from build123d import *

# Parameters (mm, degrees)
BOSS_EXTRUDE2_DEPTH = 150
SKETCH4_W           = 110
SKETCH4_H           = 150
CUT_EXTRUDE1_DEPTH  = 150
FILLET1_R           = 5
SKETCH5_R           = 17.5
CUT_EXTRUDE2_DEPTH  = 378


with BuildPart() as part:
    # Sketch3 → Boss-Extrude2 (new, symmetric)
    with BuildSketch(Plane.XY):
        with BuildLine():
            Line((0, 0), (150, 0))
            ThreePointArc((150, 0), (188.540496218, 7.5), (150, 15))
            Line((150, 15), (0, 15))
            Line((0, 15), (0, 0))
        make_face()
    extrude(amount=BOSS_EXTRUDE2_DEPTH, both=True)

    # Sketch4 → Cut-Extrude1 (cut, symmetric)
    with BuildSketch(Plane(origin=(0, 0, 0), x_dir=(1, 0, 0), z_dir=(0, 1, 0))):
        with Locations((140, 0)):
            Rectangle(SKETCH4_W, SKETCH4_H)
    extrude(amount=CUT_EXTRUDE1_DEPTH, both=True, mode=Mode.SUBTRACT)

    # Fillet1
    fillet1_edges = [part.edges().sort_by_distance(p)[0] for p in [
        (150, 15, -112.5),
        (150, 0, -112.5),
        (85, 7.5, 75),
        (85, 7.5, -75),
        (0, 7.5, 150),
        (0, 7.5, -150),
        (150, 15, 112.5),
        (150, 0, 112.5),
    ]]
    fillet(fillet1_edges, radius=FILLET1_R)

    # Sketch5 → Cut-Extrude2 (cut, symmetric)
    with BuildSketch(Plane.XY.offset(150)):
        with Locations((168.540496218, 7.5)):
            Circle(SKETCH5_R)
    extrude(amount=CUT_EXTRUDE2_DEPTH, both=True, mode=Mode.SUBTRACT)


solid = part.part
The model under review builds one solid part; all positions refer to its coordinate system, in mm. A direction names the side the tool comes from. Coordinates: 2 decimals unless noted, no trailing zeros. Loops run counter-clockwise (first coordinate to the right, second up) from the corner with the lowest first, then second, coordinate; pieces in that order, holes last.
(1) Consider section B-B, the plane x = 157. Give the boundary of the cut face in (y, z).
Determined:
outline: (-8.83, -150) - (-5.66, -150) - (-5.66, -75) - (-8.83, -75) - close; (-8.83, 75) - (-5.66, 75) - (-5.66, 150) - (-8.83, 150) - close; (20.66, -150) - (23.83, -150) - (23.83, -75) - (20.66, -75) - close; (20.66, 75) - (23.83, 75) - (23.83, 150) - (20.66, 150) - close
(2) Consider section C-C, the plane x = 97. Give the boundary of the cut face in (y, z).
Determined:
outline: (0, -150) - (15, -150) - (15, -75) - (0, -75) - close; (0, 75) - (15, 75) - (15, 150) - (0, 150) - close
(3) Consider section D-D, the plane z = 57.5. Give the boundary of the cut face in (x, y).
Determined:
outline: (0, 0) - (85, 0) - (85, 15) - (0, 15) - close
(4) Tool access review of faces 4 (the flat face through (56, 0, 2)), 5 (the flat face through (132, 6, -75)), 6 (the flat face through (58, 15, 2)), 7 (the flat face through (90, 5, 150)): name each direction out of +Z, -Z, +X, -X, +Y, -Y from which nothing blocks a thin tool from reaching the whole face with its end or side.
Determined:
face 4: +Z, -Z, -X, -Y
face 5: +X, +Y, -Y
face 6: +Z, -Z, -X, +Y
face 7: +Z, +X, -X, +Y, -Y
(5) Consider section A-A, the plane y = 7.5. Give the boundary of the cut face in (x, z), plus the area to 3 significant figures.
Determined:
outline: (0, -145) arc R5 ccw to (5, -150) - (151.04, -150) - (151.04, -75) - (90, -75) arc R5 cw to (85, -70) - (85, 70) arc R5 cw to (90, 75) - (151.04, 75) - (151.04, 150) - (5, 150) arc R5 ccw to (0, 145) - close; (186.04, -150) - (188.54, -150) - (188.54, -75) - (186.04, -75) - close; (186.04, 75) - (188.54, 75) - (188.54, 150) - (186.04, 150) - close
area: 35,800 mm2
(6) Insertion check: P1, Ø16.5, axis at y = 5, z = 25, coming from the +X side; P2, Ø3, axis at x = 23.5, z = 54, coming from the +Y side; P3, Ø10, axis at x = 150, z = -78.5, coming from the +Y side. Each pin has a flat end and moves straight along its axis. Give the tip position at first contact, or say it passes through.
Determined:
P1: stops at x = 85
P2: stops at y = 15
P3: stops at y = 22.22
(7) Wall thickness on L1, parallel to Z at x = 99.5, y = 12.5; L2, parallel to X at y = 7, z = 99; L3, parallel to Y at x = 145, z = -135.5: over which ranges is each line inside the solid? List them lowest first.
Determined:
L1: z = -150 to -75, 75 to 150
L2: x = 0 to 151.05, 186.03 to 188.53
L3: y = 0 to 15
(8) Draft analysis for pull direction Z (two halves, no side actions). For faces 1 (the flat face through (85, 8, 1)), 2 (the cylindrical face through (188.527, 6.767, 113.025)), 3 (the flat face through (90, 5, -150)), state which applies: +Z half, -Z half, draft (parallel to the pull), parting line (faces both ways), or undercut.
Determined:
face 1: undercut
face 2: draft
face 3: -Z half
